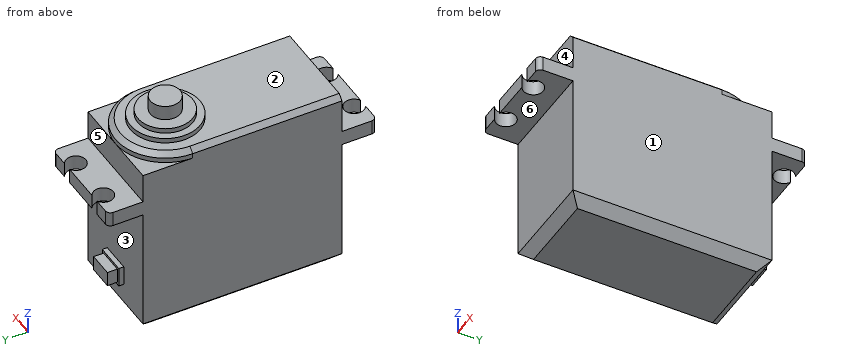
from build123d import *

# Parameters (mm, degrees)
SKETCH1_W            = 20
SKETCH1_H            = 40
BOSS_EXTRUDE1_DEPTH  = 36
CHAMFER1_SIZE        = 2
BOSS_EXTRUDE7_DEPTH  = 3
FILLET1_R            = 1
FILLET2_R            = 1
SKETCH3_W            = 6
SKETCH3_H            = 4
BOSS_EXTRUDE8_DEPTH  = 1
SKETCH4_W            = 5
SKETCH4_H            = 3
BOSS_EXTRUDE9_DEPTH  = 2
BOSS_EXTRUDE10_DEPTH = 2
CHAMFER2_SIZE        = 1
SKETCH6_R            = 7
BOSS_EXTRUDE11_DEPTH = 1
SKETCH7_R            = 5.5
BOSS_EXTRUDE12_DEPTH = 1
SKETCH8_R            = 3
BOSS_EXTRUDE13_DEPTH = 3


with BuildPart() as part:
    # Sketch1 → Boss-Extrude1 (new body)
    with BuildSketch(Plane.XY):
        Rectangle(SKETCH1_W, SKETCH1_H)
    extrude(amount=BOSS_EXTRUDE1_DEPTH)

    # Chamfer1
    chamfer1_edges = [part.edges().sort_by_distance(p)[0] for p in [
        (0, -20, 0),
        (-10, 0, 0),
        (0, 20, 0),
        (10, 0, 0),
    ]]
    chamfer(chamfer1_edges, length=CHAMFER1_SIZE)

    # Sketch2 → Boss-Extrude7 (add)
    with BuildSketch(Plane.XY.offset(27)):
        with BuildLine():
            Line((-10, 20), (10, 20))
            Line((10, 20), (10, 27))
            Line((10, 27), (5.871779789, 27))
            ThreePointArc((5.871779789, 27), (5, 23.2), (4.128220211, 27))
            Line((4.128220211, 27), (-4.128220211, 27))
            ThreePointArc((-4.128220211, 27), (-5, 23.2), (-5.871779789, 27))
            Line((-5.871779789, 27), (-10, 27))
            Line((-10, 27), (-10, 20))
        make_face()
    boss_extrude7 = extrude(amount=BOSS_EXTRUDE7_DEPTH)

    # Fillet1
    fillet1_edges = [part.edges().sort_by_distance(p)[0] for p in [
        (10, 27, 28.5),
        (-10, 27, 28.5),
    ]]
    fillet(fillet1_edges, radius=FILLET1_R)

    # Mirror1: Boss-Extrude7 across plane
    add(boss_extrude7.mirror(Plane.ZX))

    # Fillet2
    fillet2_edges = [part.edges().sort_by_distance(p)[0] for p in [
        (-10, -27, 28.5),
        (10, -27, 28.5),
    ]]
    fillet(fillet2_edges, radius=FILLET2_R)

    # Sketch3 → Boss-Extrude8 (add)
    with BuildSketch(Plane(origin=(0, 20, 0), x_dir=(1, 0, 0), z_dir=(0, 1, 0))):
        with Locations((0, -8)):
            Rectangle(SKETCH3_W, SKETCH3_H)
    extrude(amount=BOSS_EXTRUDE8_DEPTH)

    # Sketch4 → Boss-Extrude9 (add)
    with BuildSketch(Plane(origin=(0, 21, 0), x_dir=(1, 0, 0), z_dir=(0, 1, 0))):
        with Locations((0.024838868, -8.004270903)):
            Rectangle(SKETCH4_W, SKETCH4_H)
    extrude(amount=BOSS_EXTRUDE9_DEPTH)

    # Sketch5 → Boss-Extrude10 (add)
    with BuildSketch(Plane.XY.offset(36)):
        with BuildLine():
            Line((-10, 10), (-10, -20))
            Line((-10, -20), (10, -20))
            Line((10, -20), (10, 10))
            ThreePointArc((10, 10), (0, 20), (-10, 10))
        make_face()
    extrude(amount=BOSS_EXTRUDE10_DEPTH)

    # Chamfer2
    chamfer2_edges = [part.edges().sort_by_distance(p)[0] for p in [
        (10, -5, 38),
        (0, 20, 38),
        (-10, -5, 38),
    ]]
    chamfer(chamfer2_edges, length=CHAMFER2_SIZE)

    # Sketch6 → Boss-Extrude11 (add)
    with BuildSketch(Plane.XY.offset(38)):
        with Locations((0, 10)):
            Circle(SKETCH6_R)
    extrude(amount=BOSS_EXTRUDE11_DEPTH)

    # Sketch7 → Boss-Extrude12 (add)
    with BuildSketch(Plane.XY.offset(39)):
        with Locations((0, 10)):
            Circle(SKETCH7_R)
    extrude(amount=BOSS_EXTRUDE12_DEPTH)

    # Sketch8 → Boss-Extrude13 (add)
    with BuildSketch(Plane.XY.offset(40)):
        with Locations((0, 10)):
            Circle(SKETCH8_R)
    extrude(amount=BOSS_EXTRUDE13_DEPTH)


solid = part.part
CAD build for the part. Positions are in the model's coordinates, mm. Face numbers are marked on the shaded views. A direction names the side the tool comes from. Give positions to 0.01 mm unless a question says otherwise; leave off trailing zeros. Loops run counter-clockwise (first coordinate to the right, second up) from the corner with the lowest first, then second, coordinate; pieces in that order, holes last. Notation, with made-up numbers: M 83.5,1.25 L 129.5,1.25 A24 ccw 129.5,25.25 Z; hole C 44.25,-24 d6. An arc over 180 degrees is marked long. Write each question's results on one line, items separated by ' | '.
Q1. Mould opens along Z. For the marked faces 1, 2 and 3 say: pulls with the +Z half, pulls with the -Z half, needs draft (parallel to the pull), parting line crosses it, or undercut.
Geometry check:
face 1: needs draft | face 2: pulls with the +Z half | face 3: undercut
Q2. Band-saw the part on A-A on z = 8. Write the cut outline in (x, y), and give its area (3 significant figures).
Geometry check:
outline: M -10,-20 L 10,-20 L 10,20 L 3,20 L 3,21 L 2.52,21 L 2.52,23 L -2.48,23 L -2.48,21 L -3,21 L -3,20 L -10,20 Z | area: 816 mm²
Q3. Band-saw the part on B-B on y = -10.5. Write the cut outline in (x, z), and give its area (3 significant figures).
Geometry check:
outline: M -10,2 L -8,0 L 8,0 L 10,2 L 10,37 L 9,38 L -9,38 L -10,37 Z | area: 755 mm²
Q4. Which spindle directions (+Z, -Z, +X, -X, +Y, -Y) get a long thin tool onto all of the face, cutting with end or side? Do the marked faces 4, 5 and 6. Say none if no direction does.
Geometry check:
face 4: +Z, +X, -X, -Y | face 5: +Z, +X, -X, +Y | face 6: -Z, +X, -X, -Y
Q5. Flat gauge pins, fed straight in: P1, Ø6, axis at x = 1.5, z = 16, coming from the +Y side; P2, Ø3.5, axis at x = -1.5, y = -23, coming from the +Z side; P3, Ø5.5, axis at x = 0.5, y = 22, coming from the -Z side; P4, Ø2.5, axis at x = 5, y = -25.2, coming from the +Z side. Where does each tip first touch, or does it go through?
Geometry check:
P1: stops at y = 20 | P2: stops at z = 30 | P3: stops at z = 1.25 | P4: passes through
Q6. Band-saw the part on C-C on y = 5.5. Write the cut outline in (x, z).
Geometry check:
outline: M -10,2 L -8,0 L 8,0 L 10,2 L 10,37 L 9,38 L 5.36,38 L 5.36,39 L 3.16,39 L 3.16,40 L -3.16,40 L -3.16,39 L -5.36,39 L -5.36,38 L -9,38 L -10,37 Z
Q7. Probe probe 1 along X at (y, z) = (-25.2, 27.9); probe 2 along Y at (x, z) = (-8.5, 23.5); probe 3 along Y at (x, z) = (-5, 28.1). List the from-to ranges inside material, lowest first.
Geometry check:
probe 1: x = -10 to -7, -3 to 3, 7 to 10 | probe 2: y = -20 to 20 | probe 3: y = -23.2 to 23.2
